```python
from build123d import *

# Parameters (mm, degrees)
BOSS_EXTRUDE1_DEPTH = 5
SKETCH2_W           = 20.5
SKETCH2_H           = 30
SKETCH2_R           = 2.5
BOSS_EXTRUDE2_DEPTH = 5
FILLET1_R           = 10.25


with BuildPart() as part:
    # Sketch1 → Boss-Extrude1 (new body)
    with BuildSketch(Plane(origin=(0, 0, 0), x_dir=(1, 0, 0), z_dir=(0, 1, 0))):
        Polygon((44.375484097, 7.788988346), (75.375484097, 7.788988346), (80.375484097, 7.788988346), (80.375484097, 12.788988346), (75.375484097, 12.788988346), (75.375484097, 18.288988346), (73.375484097, 18.288988346), (73.375484097, 17.188988346), (71.075484097, 17.188988346), (71.075484097, 18.288988346), (68.375484097, 18.288988346), (68.375484097, 21.288988346), (71.075484097, 21.288988346), (71.075484097, 22.388988346), (73.375484097, 22.388988346), (73.375484097, 21.288988346), (75.375484097, 21.288988346), (75.375484097, 26.788988346), (80.375484097, 26.788988346), (80.375484097, 31.788988346), (75.375484097, 31.788988346), (44.375484097, 31.788988346), (39.375484097, 31.788988346), (39.375484097, 26.788988346), (44.375484097, 26.788988346), (44.375484097, 21.288988346), (46.375484097, 21.288988346), (46.375484097, 22.388988346), (48.675484097, 22.388988346), (48.675484097, 21.288988346), (51.375484097, 21.288988346), (51.375484097, 18.288988346), (48.675484097, 18.288988346), (48.675484097, 17.188988346), (46.375484097, 17.188988346), (46.375484097, 18.288988346), (44.375484097, 18.288988346), (44.375484097, 12.788988346), (39.375484097, 12.788988346), (39.375484097, 7.788988346), align=None)
    extrude(amount=BOSS_EXTRUDE1_DEPTH)

    # Sketch2 → Boss-Extrude2 (add)
    with BuildSketch(Plane(origin=(0, 5, 0), x_dir=(1, 0, 0), z_dir=(0, 1, 0))):
        with Locations((59.875484097, -7.211011654)):
            Rectangle(SKETCH2_W, SKETCH2_H)
        with Locations(Location((59.875484097, -11.961011654, 0), (0, 0, 270))):
            Circle(SKETCH2_R, mode=Mode.SUBTRACT)
    extrude(amount=-BOSS_EXTRUDE2_DEPTH)

    # Fillet1
    fillet1_edges = [part.edges().sort_by_distance(p)[0] for p in [
        (49.625484097, 2.5, 22.211011654),
        (70.125484097, 2.5, 22.211011654),
    ]]
    fillet(fillet1_edges, radius=FILLET1_R - 0.0001)  # a hair under: the kernel refuses the full size


solid = part.part
```
For this review, take the finished solid that the model builds, in its own axes (mm). A direction names the side the tool comes from. Round coordinates to 2 decimals unless told otherwise and drop trailing zeros. Order: outer loops, then holes, each group sorted by start corner. A loop starts at its lowest first (then second) coordinate and runs counter-clockwise, first axis right, second up. Notation, with made-up numbers: (-28, 48.5) -> (14, 48.5) arc R37 cw to (14, 85.5) -> close; hole circle Ø7 at (70, 75.25). An arc over 180 degrees is marked (long way). Use a Markdown table: item, result.
Item 1: Machinability: for faces 4 (the flat face through (60, 2, -31.789)), 5 (the flat face through (78, 2, -12.789)), 6 (the flat face through (51.375, 2, -20)), 7 (the flat face through (73.375, 2, -18)), which of the approach directions +Z, -Z, +X, -X, +Y, -Y give a long, thin tool a straight path to every point of the face, cutting with its end or side? Answer none if there is none.
Resolved:
| item | result |
|---|---|
| face 4 | -Z, +X, -X, +Y, -Y |
| face 5 | +X, +Y, -Y |
| face 6 | -X, +Y, -Y |
| face 7 | +Y, -Y |
Item 2: For line 1 along X through (y, z) = (0.4, -18); line 2 along Z through (x, y) = (46.5, 0.9); line 3 along X through (y, z) = (3.75, 1), list the stretches that pass through material, from the lowest coordinate up. Write a range as [from, to].
Resolved:
| item | result |
|---|---|
| line 1 | x = [44.38, 46.38], [48.68, 71.08], [73.38, 75.38] |
| line 2 | z = [-31.79, -22.39], [-17.19, -7.79] |
| line 3 | x = [49.63, 70.13] |
Item 3: Take a section at D-D (x = 52.5). State the section outline as (y, z) points.
Resolved:
| item | result |
|---|---|
| outline | (0, -31.79) -> (5, -31.79) -> (5, 19.08) -> (0, 19.08) -> close |
Item 4: For pin 1 (0.9 mm diameter, centred on y = 3.5, z = -17.5, fed in from +X); pin 2 (0.6 mm diameter, centred on y = 2.5, z = -18, fed in from -X); pin 3 (1.6 mm diameter, centred on x = 74.5, y = 3.5, fed in from +Z), all flat-tipped, find the tip position at first contact; note any pin that passes through.
Resolved:
| item | result |
|---|---|
| pin 1 | stops at x = 75.38 |
| pin 2 | stops at x = 44.38 |
| pin 3 | stops at z = -7.79 |
Item 5: Take a section at A-A (x = 42). State the section outline as (y, z) points, plus the area to 3 significant figures.
Resolved:
| item | result |
|---|---|
| outline | (0, -31.79) -> (5, -31.79) -> (5, -26.79) -> (0, -26.79) -> close; (0, -12.79) -> (5, -12.79) -> (5, -7.79) -> (0, -7.79) -> close |
| area | 50.0 mm² |
Item 6: Take a section at B-B (z = 13.5). State the section outline as (x, y) points.
Resolved:
| item | result |
|---|---|
| outline | (49.74, 0) -> (57.91, 0) -> (57.91, 5) -> (49.74, 5) -> close; (61.85, 0) -> (70.01, 0) -> (70.01, 5) -> (61.85, 5) -> close |
Item 7: Take a section at C-C (z = -16). State the section outline as (x, y) points.
Resolved:
| item | result |
|---|---|
| outline | (44.38, 0) -> (75.38, 0) -> (75.38, 5) -> (44.38, 5) -> close |
Item 8: Draft analysis for pull direction Z (two halves, no side actions). For faces 1 (the flat face through (44, 2, -7.789)), 2 (the flat face through (80.375, 2, -29)), 3 (the flat face through (68.375, 2, -20)), state which applies: +Z half, -Z half, draft (parallel to the pull), parting line (faces both ways), or undercut.
Resolved:
| item | result |
|---|---|
| face 1 | +Z half |
| face 2 | draft |
| face 3 | undercut |
